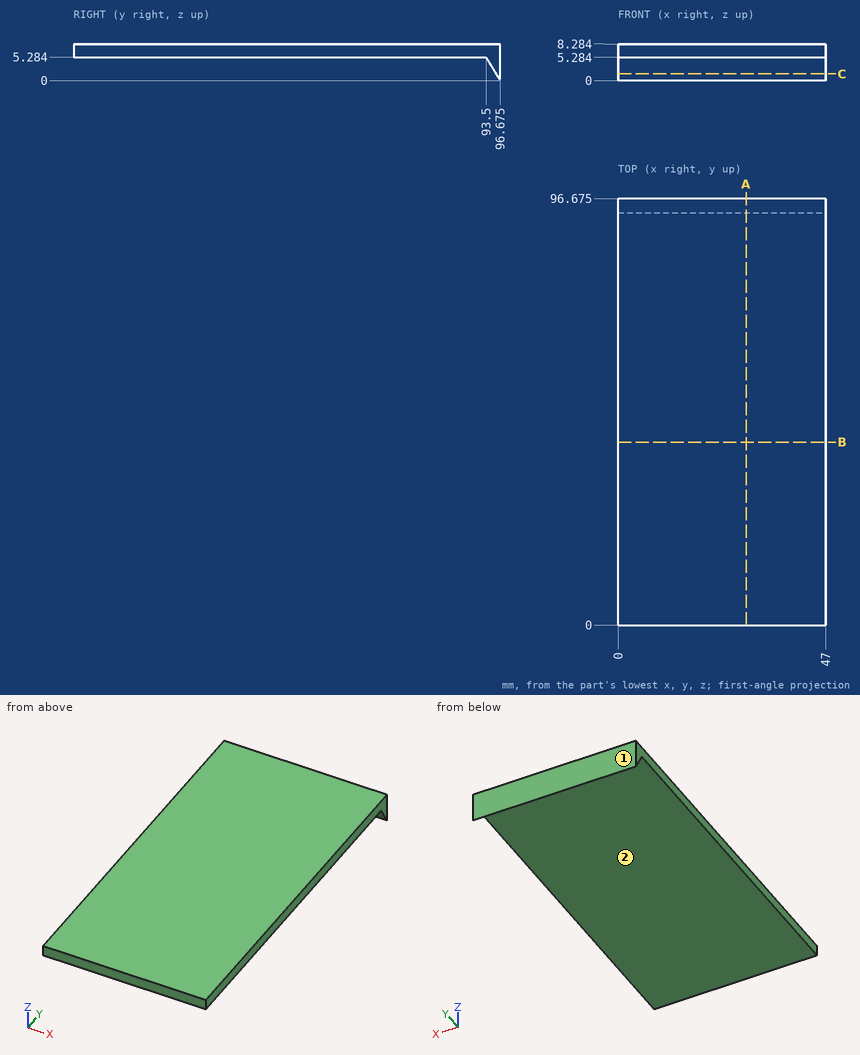
Print and shaded views of the part. All mm, measured from the part's lowest x, y and z. A direction names the side the tool comes from. Round coordinates to 2 decimals unless told otherwise and drop trailing zeros. Loops run counter-clockwise (first coordinate to the right, second up) from the corner with the lowest first, then second, coordinate; pieces in that order, holes last. Notation, with made-up numbers: (43, 65) -> (56, 65) arc R27 cw to (56, 94) -> close; hole circle Ø1 at (-2.5, -25). An arc over 180 degrees is marked (long way). Use CSV: the item, a comma, the result in double quotes. Start each with the question number.
1) Cut at C-C, the plane z = 1.5. Write the cut outline in (x, y) (3 decimals).
2) Which spindle directions (+Z, -Z, +X, -X, +Y, -Y) get a long thin tool onto all of the face, cutting with end or side? Do the marked faces 1 and 2. Say none if no direction does.
3) Cut at A-A, the plane x = 29. Write the cut outline in (y, z) (3 decimals).
4) Drop flat-ended pins along their axis: P1, Ø23.5, axis at x = 29.5, y = 47, coming from the -Z side; P2, Ø1.5, axis at y = 26.5, z = 4.5, coming from the -X side. Give the stop position or say it passes through.
5) Cut at B-B, the plane y = 41.5. Write the cut outline in (x, z), plus the area to 3 significant figures.
6) Wall check: L1, parallel to Z at x = 33, y = 61; L2, parallel to Y at x = 10, z = 3.25 (1 decimal); L3, parallel to Y at x = 12, z = 3.5 (3 decimals). Give the ranges that are in metal, low to high. Write a range as [from, to].
Determined:
1,outline,"(0, 95.774) -> (47, 95.774) -> (47, 96.675) -> (0, 96.675) -> close"
2,face 1,"+Z, -Z, +X, -X, +Y"
2,face 2,"-Z, +X, -X, -Y"
3,outline,"(0, 5.284) -> (93.5, 5.284) -> (96.675, 0) -> (96.675, 8.284) -> (0, 8.284) -> close"
4,P1,"stops at z = 5.28"
4,P2,"passes through"
5,outline,"(0, 5.28) -> (47, 5.28) -> (47, 8.28) -> (0, 8.28) -> close"
5,area,"141 mm2"
6,L1,"z = [5.28, 8.28]"
6,L2,"y = [94.7, 96.7]"
6,L3,"y = [94.572, 96.675]"
